from build123d import *

# Parameters (mm, degrees)
BOSS_EXTRUDE1_DEPTH      = 2
SKETCH1_3_W              = 10
SKETCH1_3_H              = 4.75
BOSS_EXTRUDE2_DEPTH      = 12.7
BOSS_EXTRUDE3_START      = 12.7
SKETCH3_W                = 11.9
SKETCH3_H                = 4.75
SKETCH3_W_2              = 10.75
BOSS_EXTRUDE3_DEPTH      = 12.7
BOSS_EXTRUDE4_START      = 25.4
SKETCH3_3_W              = 11.9
SKETCH3_3_H              = 4.75
SKETCH3_3_W_2            = 10.75
SKETCH3_3_W_3            = 1.15
BOSS_EXTRUDE4_DEPTH      = 2
CUT_EXTRUDE1_START       = -1.1
SKETCH2_R                = 1.2
CUT_EXTRUDE1_DEPTH       = 8
CUT_EXTRUDE2_START       = 3.1
SKETCH2_3_R              = 1.2
CUT_EXTRUDE2_DEPTH       = 8
BOSS_EXTRUDE5_START      = 17
SKETCH1_4_W              = 7.7
SKETCH1_4_H              = 6.8
SKETCH1_4_R              = 1.7
BOSS_EXTRUDE5_DEPTH      = 3
FILLET1_R                = 2
CUT_EXTRUDE3_START       = 12.7
SKETCH5_W                = 14.55
SKETCH5_H                = 4.75
CUT_EXTRUDE3_DEPTH       = 2
CUT_EXTRUDE4_START       = 12.7
SKETCH6_W                = 7.7
SKETCH6_H                = 4.75
CUT_EXTRUDE4_DEPTH       = 4
BOSS_EXTRUDE6_DEPTH      = 2
BOSS_EXTRUDE6_DEPTH_BACK = 2
BOSS_EXTRUDE6_START      = 27.4
SKETCH7_W                = 9.1
SKETCH7_H                = 5
SKETCH7_R                = 1.2
SKETCH7_W_2              = 4
SKETCH7_H_2              = 15


with BuildPart() as part:
    # Sketch1 → Boss-Extrude1 (new body)
    with BuildSketch(Plane(origin=(0, 0, 0), x_dir=(1, 0, 0), z_dir=(0, 1, 0))):
        Polygon((-1.1, 16.25), (-1.1, -16.25), (8.9, -16.25), (8.9, -11.5), (17.65, -11.5), (17.65, 16.25), align=None)
    extrude(amount=-BOSS_EXTRUDE1_DEPTH)

    # Sketch1<3> → Boss-Extrude2 (add)
    with BuildSketch(Plane(origin=(0, 0, 0), x_dir=(1, 0, 0), z_dir=(0, 1, 0))):
        Polygon((5.45, 16.25), (-1.1, 16.25), (-1.1, 11.5), (17.65, 11.5), (17.65, 16.25), align=None)
        with Locations((3.9, -13.875)):
            Rectangle(SKETCH1_3_W, SKETCH1_3_H)
    extrude(amount=BOSS_EXTRUDE2_DEPTH)

    # Sketch3 → Boss-Extrude3 (add)
    with BuildSketch(Plane(origin=(0, 0, 0), x_dir=(1, 0, 0), z_dir=(0, 1, 0)).offset(BOSS_EXTRUDE3_START)):
        with Locations((-2.85, 13.875)):
            Rectangle(SKETCH3_W, SKETCH3_H)
        with Locations((-2.275, -13.875)):
            Rectangle(SKETCH3_W_2, SKETCH3_H)
    extrude(amount=BOSS_EXTRUDE3_DEPTH)

    # Sketch3<3> → Boss-Extrude4 (add)
    with BuildSketch(Plane(origin=(0, 0, 0), x_dir=(1, 0, 0), z_dir=(0, 1, 0)).offset(BOSS_EXTRUDE4_START)):
        with Locations((-2.85, 13.875)):
            Rectangle(SKETCH3_3_W, SKETCH3_3_H)
        Polygon((3.1, -11.5), (3.1, 11.5), (-8.8, 11.5), (-8.8, -11.5), (-7.65, -11.5), align=None)
        with Locations((-2.275, -13.875)):
            Rectangle(SKETCH3_3_W_2, SKETCH3_3_H)
        with Locations((-8.225, -13.875)):
            Rectangle(SKETCH3_3_W_3, SKETCH3_3_H)
    extrude(amount=BOSS_EXTRUDE4_DEPTH)

    # Sketch2 → Cut-Extrude1 (cut)
    with BuildSketch(Plane(origin=(0, 0, 0), x_dir=(0, 0, -1), z_dir=(1, 0, 0)).offset(CUT_EXTRUDE1_START)):
        with Locations(Location((-13.7, 6.45, 0), (0, 0, 180))):
            Circle(SKETCH2_R)
        with Locations(Location((13.7, 6.45, 0), (0, 0, 180))):
            Circle(SKETCH2_R)
    extrude(amount=CUT_EXTRUDE1_DEPTH, mode=Mode.SUBTRACT)

    # Sketch2<3> → Cut-Extrude2 (cut)
    with BuildSketch(Plane(origin=(0, 0, 0), x_dir=(0, 0, -1), z_dir=(1, 0, 0)).offset(CUT_EXTRUDE2_START)):
        with Locations(Location((13.7, 19.15, 0), (0, 0, 180))):
            Circle(SKETCH2_3_R)
        with Locations(Location((-13.7, 19.15, 0), (0, 0, 180))):
            Circle(SKETCH2_3_R)
    extrude(amount=-CUT_EXTRUDE2_DEPTH, mode=Mode.SUBTRACT)

    # Sketch1<4> → Boss-Extrude5 (add)
    # profile 1 of 2: a face of its own
    with BuildSketch(Plane(origin=(0, 0, 0), x_dir=(1, 0, 0), z_dir=(0, 1, 0)).offset(BOSS_EXTRUDE5_START)):
        with Locations((1.6, 19.65)):
            Rectangle(SKETCH1_4_W, SKETCH1_4_H)
        with Locations(Location((1.6, 19.85, 0), (0, 0, 270))):
            Circle(SKETCH1_4_R, mode=Mode.SUBTRACT)
    # profile 2 of 2: a face of its own
    with BuildSketch(Plane(origin=(0, 0, 0), x_dir=(1, 0, 0), z_dir=(0, 1, 0)).offset(BOSS_EXTRUDE5_START)):
        with Locations((-7.8, -19.65)):
            Rectangle(SKETCH1_4_W, SKETCH1_4_H)
        with Locations(Location((-7.8, -19.85, 0), (0, 0, 270))):
            Circle(SKETCH1_4_R, mode=Mode.SUBTRACT)
    extrude(amount=-BOSS_EXTRUDE5_DEPTH)

    # Fillet1
    fillet1_edges = [part.edges().sort_by_distance(p)[0] for p in [
        (3.9, -2, 16.25),
        (-2.85, 27.4, 16.25),
        (8.275, -2, -16.25),
        (-2.85, 27.4, -16.25),
    ]]
    fillet(fillet1_edges, radius=FILLET1_R)

    # Sketch5 → Cut-Extrude3 (cut)
    with BuildSketch(Plane(origin=(0, 0, 0), x_dir=(1, 0, 0), z_dir=(0, 1, 0)).offset(CUT_EXTRUDE3_START)):
        with Locations((10.375, 13.875)):
            Rectangle(SKETCH5_W, SKETCH5_H)
    extrude(amount=-CUT_EXTRUDE3_DEPTH, mode=Mode.SUBTRACT)

    # Sketch6 → Cut-Extrude4 (cut)
    with BuildSketch(Plane(origin=(0, 0, 0), x_dir=(1, 0, 0), z_dir=(0, 1, 0)).offset(CUT_EXTRUDE4_START)):
        with Locations((-4.95, 13.875)):
            Rectangle(SKETCH6_W, SKETCH6_H)
    extrude(amount=CUT_EXTRUDE4_DEPTH, mode=Mode.SUBTRACT)

    # Sketch7 → Boss-Extrude6 (add, two sides: drawn at the far end of the back side and taken through both)
    # profile 1 of 3: a face of its own
    with BuildSketch(Plane(origin=(0, 0, 0), x_dir=(1, 0, 0), z_dir=(0, 1, 0)).offset(BOSS_EXTRUDE6_START - BOSS_EXTRUDE6_DEPTH_BACK)):
        with Locations((3.55, 11.43)):
            Rectangle(SKETCH7_W, SKETCH7_H)
        with Locations(Location((5.6, 11.43, 0), (0, 0, 90))):
            Circle(SKETCH7_R, mode=Mode.SUBTRACT)
    # profile 2 of 3: a face of its own
    with BuildSketch(Plane(origin=(0, 0, 0), x_dir=(1, 0, 0), z_dir=(0, 1, 0)).offset(BOSS_EXTRUDE6_START - BOSS_EXTRUDE6_DEPTH_BACK)):
        with Locations((-3, 0)):
            Rectangle(SKETCH7_W_2, SKETCH7_H_2)
    # profile 3 of 3: a face of its own
    with BuildSketch(Plane(origin=(0, 0, 0), x_dir=(1, 0, 0), z_dir=(0, 1, 0)).offset(BOSS_EXTRUDE6_START - BOSS_EXTRUDE6_DEPTH_BACK)):
        with Locations((3.55, -11.43)):
            Rectangle(SKETCH7_W, SKETCH7_H)
        with Locations(Location((5.6, -11.43, 0), (0, 0, 90))):
            Circle(SKETCH7_R, mode=Mode.SUBTRACT)
    extrude(amount=BOSS_EXTRUDE6_DEPTH + BOSS_EXTRUDE6_DEPTH_BACK)


solid = part.part
Source: CAD feature listing. Evaluate the final solid. Frame: model axes, mm. A direction names the side the tool comes from. Give positions to 0.01 mm unless a question says otherwise; leave off trailing zeros. Write each loop counter-clockwise with the first axis right and the second up, starting at its lowest first coordinate (ties: lowest second). Pieces come first, ordered by that corner, then holes. Notation, with made-up numbers: M 86,82.5 L 120,82.5 A33 cw 120,115.5 Z; hole C 23,86 d11. An arc over 180 degrees is marked long. Return JSON: item names as keys, results as strings. Group by question number.
1) Cut plane B-B, the plane y = 10. Output: boundary loops of the cut face in (x, z), plus the area to 3 significant figures.
2) Pin query (flat end, axial travel): P1, Ø4.5, axis at x = -7.8, z = 19.85, coming from the +Y side; P2, Ø2, axis at y = 26.5, z = 0, coming from the +X side; P3, Ø3, axis at y = 6.45, z = 13.7, coming from the -X side; P4, Ø10, axis at x = -3, z = -12.5, coming from the +Y side. Return the tip coordinate at first contact, or that it passes through.
3) Cut plane D-D, the plane x = 10. Output: boundary loops of the cut face in (y, z), plus the area to 3 significant figures.
4) Cut plane A-A, the plane x = 1.6. Give the number of separate pieces and of enclosed holes in the cut face, plus the area to 3 significant figures.
5) Set-up query: faces 4 (the face through (3.1, 26, 0)), 5 (the face through (-4.9, 19, -14)), 6 (the face through (4, 16, -16.25)), 7 (the face through (-2, 15, -16.25)). Return all of +Z, -Z, +X, -X, +Y, -Y with unobstructed straight access to the full face (end or side cutting, diameter ignored); none if empty.
6) Pull-direction query (Y, two-part tool) for faces 1 (the face through (-8, 17, 18)), 2 (the face through (2.84, 6.91, -12.59)), 3 (the face through (-3.95, 16, 20)); classes: pulls with the +Y half, pulls with the -Y half, needs draft (parallel to the pull), parting line crosses it, or undercut.
7) Cut plane C-C, the plane y = 15. Output: boundary loops of the cut face in (x, z).
8) Material intervals for line 1 along Z through (x, y) = (3, 6.45); line 2 along X through (y, z) = (26.4, 11.43); line 3 along Y through (x, z) = (0.5, -13.7), sorted ascending. Write a range as [from, to].
Recorded:
{
 "1": {"outline": "M -1.1,-16.25 L 17.65,-16.25 L 17.65,-11.5 L -1.1,-11.5 Z; M -1.1,11.5 L 8.9,11.5 L 8.9,16.25 L -1.1,16.25 Z", "area": "137 mm²"},
 "2": {"P1": "stops at y = 17", "P2": "stops at x = 3.1", "P3": "stops at x = -1.1", "P4": "stops at y = 29.4"},
 "3": {"outline": "M -2,-14.25 A2 ccw 0,-16.25 L 10.7,-16.25 L 10.7,-11.5 L 0,-11.5 L 0,11.5 L -2,11.5 Z", "area": "105 mm²"},
 "4": {"separate pieces": "2", "enclosed holes": "5", "area": "380 mm²"},
 "5": {"face 4": "+X, +Y", "face 5": "+X", "face 6": "+Z, +X, +Y", "face 7": "-X, -Y"},
 "6": {"face 1": "pulls with the +Y half", "face 2": "undercut", "face 3": "needs draft"},
 "7": {"outline": "M -11.65,16.25 L -7.65,16.25 L -7.65,11.5 L 3.1,11.5 L 3.1,16.25 L -3.95,16.25 L -3.95,23.05 L -11.65,23.05 Z; M -2.25,-23.05 L 5.45,-23.05 L 5.45,-16.25 L 3.1,-16.25 L 3.1,-11.5 L -1.1,-11.5 L -1.1,-16.25 L -2.25,-16.25 Z; hole C -7.8,19.85 d3.4; hole C 1.6,-19.85 d3.4"},
 "8": {"line 1": "z = [-16.25, -14.9], [-12.5, -11.5], [11.5, 12.5], [14.9, 16.25]", "line 2": "x = [-8.8, 4.4], [6.8, 8.1]", "line 3": "y = [-2, 5.25], [7.65, 17.95], [20.35, 29.4]"}
}
